Design review of the part built by this model. Coordinates are the model's own, in mm. Give positions to 0.01 mm unless a question says otherwise; leave off trailing zeros. Loops run counter-clockwise (first coordinate to the right, second up) from the corner with the lowest first, then second, coordinate; pieces in that order, holes last. Notation, with made-up numbers: M 70,-15.5 L 74,-15.5 A20 cw 74,22.5 Z; hole C 73,12.5 d6. An arc over 180 degrees is marked long. Use CSV: the item, a comma, the result in double quotes.
from build123d import *

# Parameters (mm, degrees)
F0_R     = 2.78
F1_DEPTH = 45
F2_R     = 2.701299
F3_DEPTH = 44.35984
F4_R     = 1.253885
F5_DEPTH = 0.25
F6_R     = 0.107264


with BuildPart() as f1:
    # F0 (on Top) → F1 (new body)
    with BuildSketch(Plane.XY):
        Circle(F0_R)
    extrude(amount=F1_DEPTH)

    # F2 (on face) → F3 (cut)
    with BuildSketch(Plane.XY.offset(45)):
        Circle(F2_R)
    extrude(amount=-F3_DEPTH, mode=Mode.SUBTRACT)

    # F4 (on face) → F5 (cut)
    with BuildSketch(Plane(origin=(0, 0, 0), x_dir=(1, 0, 0), z_dir=(0, 0, -1))):
        Circle(F4_R)
    extrude(amount=-F5_DEPTH, mode=Mode.SUBTRACT)

    # F6
    f6_edges = [f1.edges().sort_by_distance(p)[0] for p in [
        (-1.253885, 0, 0.25),
    ]]
    fillet(f6_edges, radius=F6_R)


solid = f1.part
(1) We need section D-D on y = -2.05. State the section outline as (x, z) points, then the cut area to 3 significant figures.
A:
outline,"M -1.88,0 L 1.88,0 L 1.88,45 L 1.76,45 L 1.76,0.64 L -1.76,0.64 L -1.76,45 L -1.88,45 Z"
area,"12.9 mm²"
(2) We need section A-A on y = 0. State the section outline as (x, z) points.
A:
outline,"M -2.78,0 L -1.25,0 L -1.25,0.14 A0.11 cw -1.15,0.25 L 1.15,0.25 A0.11 cw 1.25,0.14 L 1.25,0 L 2.78,0 L 2.78,45 L 2.7,45 L 2.7,0.64 L -2.7,0.64 L -2.7,45 L -2.78,45 Z"
(3) Clearance check with flat-ended pins moving along their axes: P1, Ø2.5, axis at x = 0, y = 0, coming from the +Z side; P2, Ø1.1, axis at x = 0.5, y = 0, coming from the -Z side; P3, Ø2, axis at y = -1.5, z = 35.5, coming from the -X side. State where each tip first meets the part, or that it passes through.
A:
P1,"z = 0.64"
P2,"z = 0.25"
P3,"x = -2.73"
(4) Wall thickness on line 1 along Y through (x, z) = (0, 0.15); line 2 along Z through (x, y) = (2, 0.05); line 3 along X through (y, z) = (2.45, 31): over which ranges is each line inside the solid? List them lowest first. Write a range as [from, to].
A:
line 1,"[-2.78, -1.25], [1.25, 2.78]"
line 2,"[0, 0.64]"
line 3,"[-1.31, -1.14], [1.14, 1.31]"
(5) We need section B-B on z = 14.5. State the section outline as (x, y) points.
A:
outline,"C 0,0 d5.56; hole C 0,0 d5.4"
(6) The part is to be moulded in two halves that separate along Y. For faces 1 (the flat face through (0, 0, 0.64)), 2 (the flat face through (1, -1, 0)), say which applies: released by +Y, released by -Y, zero draft, split by the parting line, or undercut.
A:
face 1,"undercut"
face 2,"zero draft"
